Geometry check sheet. Reference: the model listing, model coordinates, mm. Face numbers are marked on the shaded views. Give positions to 0.01 mm unless a question says otherwise; leave off trailing zeros. Order: outer loops, then holes, each group sorted by start corner. A loop starts at its lowest first (then second) coordinate and runs counter-clockwise, first axis right, second up. Notation, with made-up numbers: M 1.25,15 L 13.25,15 A32 cw 13.25,49 Z; hole C 65,30 d11. An arc over 180 degrees is marked long. Put each result on its own line as item: value. Start each with the question number.
Q1. Mould release check, pull along X, two halves, no side actions. Record for the marked faces 1, 2 and 3: +X half, -X half, draft (parallel to the pull), parting line (faces both ways), or undercut.
Q2. Section check A-A on y = -15.5. Record the cut outline in (x, z), then the cut area to 3 significant figures.
Q3. Section check C-C on x = 0. Record the cut outline in (y, z).
Q4. Material ranges on L1, parallel to Y at x = -15.5, z = 9.75; L2, parallel to Y at x = 0, z = 6.25; L3, parallel to X at y = -8, z = 10, recorded low to high.
Autodesk Inventor part; units mm, degrees
sketch "Эскиз1" plane through (0, 0, 0) normal (0, 0, 1) x (1, 0, 0)
  line L0 (21, -21) -> (-21, -21)
  line L1 (-21, -21) -> (-21, 21)
  line L2 (-21, 21) -> (21, 21)
  line L3 (21, 21) -> (21, -21)
  line L4 (21, -21) -> (-21, 21) construction
  line L5 (-21, -21) -> (21, 21) construction
  point P0 (0, 0)
  dimension "d0" = 42
extrude "Выдавливание1" add sketch "Эскиз1" along normal blind 12
sketch "Эскиз2" plane through (0, 0, 12) normal (0, 0, 1) x (1, 0, 0)
  circle A0 centre (0, 0) radius 11.6
  dimension "d3" = 23.2
extrude "Выдавливание2" cut sketch "Эскиз2" against normal up to next
sketch "Эскиз3" plane through (0, 0, 12) normal (0, 0, 1) x (1, 0, 0)
  circle A0 centre (-15.5, 15.5) radius 1.35
  circle A1 centre (15.5, 15.5) radius 1.35
  circle A2 centre (-15.5, -15.5) radius 1.35
  circle A3 centre (15.5, -15.5) radius 1.35
  line L0 (-15.5, 15.5) -> (-15.5, -15.5) construction
  line L1 (-15.5, -15.5) -> (15.5, -15.5) construction
  line L2 (15.5, -15.5) -> (15.5, 15.5) construction
  line L3 (15.5, 15.5) -> (-15.5, 15.5) construction
  line L4 (-15.5, 15.5) -> (15.5, -15.5) construction
  line L5 (15.5, 15.5) -> (-15.5, -15.5) construction
  point P0 (0, 0)
  point P1 (0, 0)
  dimension "d6" = 2.7
  dimension "d7" = 31
extrude "Выдавливание3" cut sketch "Эскиз3" against normal up to next
properties part number "Крепление_мотора_V2"
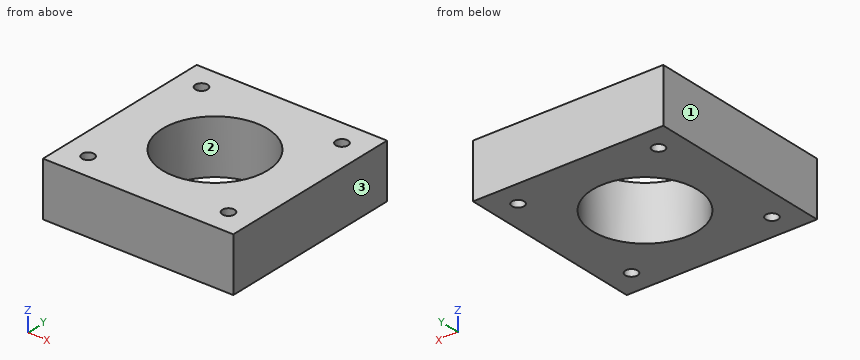
Results found:
1. face 1: -X half
1. face 2: undercut
1. face 3: +X half
2. outline: M -21,0 L -16.85,0 L -16.85,12 L -21,12 Z; M -14.15,0 L 14.15,0 L 14.15,12 L -14.15,12 Z; M 16.85,0 L 21,0 L 21,12 L 16.85,12 Z
2. area: 439 mm^2
3. outline: M -21,0 L -11.6,0 L -11.6,12 L -21,12 Z; M 11.6,0 L 21,0 L 21,12 L 11.6,12 Z
4. L1: y = -21 to -16.85, -14.15 to 14.15, 16.85 to 21
4. L2: y = -21 to -11.6, 11.6 to 21
4. L3: x = -21 to -8.4, 8.4 to 21
